from build123d import *

# Parameters (mm, degrees)
F1_DEPTH  = 25
F1_FACE_W = 66.04
F1_FACE_H = 25
F2_DEPTH  = 1.588
F2_TAPER  = -3


with BuildPart() as f1:
    # F0 (on Top) → F1 (new body)
    with BuildSketch(Plane.XY):
        Polygon((32.4131661011, 23.9884992057), (-33.6268338989, 23.9884992057), (-33.6268338989, -29.3515007943), (32.4131661011, -29.3515007943), (32.4131661011, -22.7092797923), (34.5588182305, -21.1252766549), (34.5588182305, 18.2884992057), (32.4131661011, 20.4341513352), align=None)
    extrude(amount=F1_DEPTH)

    # F1_face (on face) → F2 (join)
    with BuildSketch(Plane(origin=(-0.6068338989, -29.3515007943, 12.5), x_dir=(1, 0, 0), z_dir=(0, -1, 0))):
        Rectangle(F1_FACE_W, F1_FACE_H)
    extrude(amount=F2_DEPTH, taper=F2_TAPER)


solid = f1.part
Read the model definition and answer for the solid it produces. Units are mm, in the model's axes. A direction names the side the tool comes from. Round coordinates to 2 decimals unless told otherwise and drop trailing zeros. Write each loop counter-clockwise with the first axis right and the second up, starting at its lowest first coordinate (ties: lowest second). Pieces come first, ordered by that corner, then holes.
1. Given pin 1 Ø1.8 at (y, z) = (22.5, 17) entering from +X; pin 2 Ø8 at (x, y) = (26.5, 14.5) entering from -Z; pin 3 Ø3 at (x, y) = (7.5, -24) entering from +Z, each flat-ended and moving along its own axis, determine where each tip first touches the part or whether it passes through.
2. Straight lines are drawn through the part: L1, parallel to Z at x = 4.5, y = 21; L2, parallel to X at y = -8, z = 8; L3, parallel to X at y = 22.5, z = 14.5. For each, find the intervals that lie inside material, in ascending order.
3. Which of the six approach directions +Z, -Z, +X, -X, +Y, -Y give full straight-line access (tool end or side, diameter ignored) to faces 1 (the face through (0, -2, 25)), 2 (the face through (32.413, -26, 12)), 3 (the face through (0, -2, 0)), 4 (the face through (-33.627, -2, 12))?
4. The part is cut by section A-A, the plane y = -24. Determine the outline of the cut face in (x, z).
Values:
1. pin 1: stops at x = 32.41
1. pin 2: stops at z = 0
1. pin 3: stops at z = 25
2. L1: z = 0 to 25
2. L2: x = -33.63 to 34.56
2. L3: x = -33.63 to 32.41
3. face 1: +Z, +X, -X, +Y
3. face 2: +Z, -Z, +X
3. face 3: -Z, +X, -X, +Y
3. face 4: +Z, -Z, -X, +Y
4. outline: (-33.63, 0) - (32.41, 0) - (32.41, 25) - (-33.63, 25) - close
